Check sheet for the modelled part. Datum: model origin and axes. Units: mm. Face numbers are marked on the shaded views. A direction names the side the tool comes from. Round coordinates to 2 decimals unless told otherwise and drop trailing zeros. Loops run counter-clockwise (first coordinate to the right, second up) from the corner with the lowest first, then second, coordinate; pieces in that order, holes last. Notation, with made-up numbers: (40.25, 75) - (64.25, 75) arc R16 ccw to (64.25, 97) - close; hole circle Ø1 at (-16, 58). An arc over 180 degrees is marked (long way). Put each result on its own line as item: value.
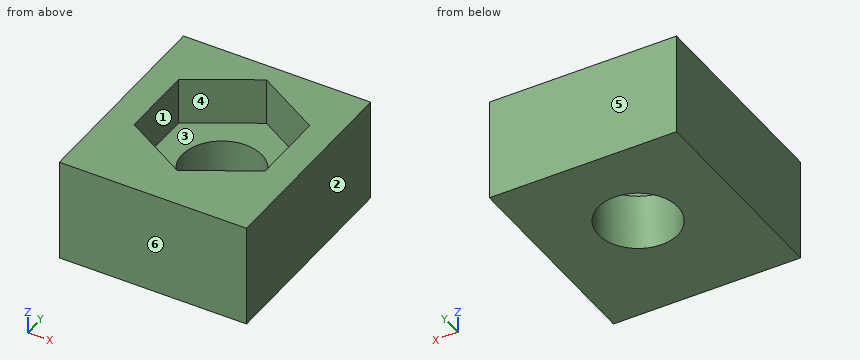
Autodesk Fusion 360 part; units mm, degrees
sketch "Sketch1" plane through (0, 0, 0) normal (0, 0, 1) x (1, 0, 0)
  line L0 (0, 0) -> (0, 8)
  line L1 (0, 0) -> (8, 0)
  line L2 (8, 0) -> (8, 8)
  line L3 (8, 8) -> (0, 8)
  dimension "d1" = 8
  dimension "d2" = 8
extrude "Extrude1" add sketch "Sketch1" along normal blind 2.4
sketch "Sketch2" plane through (0, 0, 2.4) normal (0, 0, 1) x (-1, 0, 0)
  line L0 (0, 0) -> (-8, 0)
  line L1 (-8, 0) -> (-8, -8)
  line L2 (-8, -8) -> (0, -8)
  line L3 (0, -8) -> (0, 0)
  line L4 (-8, -8) -> (0, 0)
  line L5 (-8, 0) -> (0, -8)
  line L6 (-6.8, -5.6166) -> (-4, -7.2332)
  line L7 (-4, -7.2332) -> (-1.2, -5.6166)
  line L8 (-1.2, -5.6166) -> (-1.2, -2.3834)
  line L9 (-1.2, -2.3834) -> (-4, -0.7668)
  line L10 (-4, -0.7668) -> (-6.8, -2.3834)
  line L11 (-6.8, -2.3834) -> (-6.8, -5.6166)
  point P0 (-4, -4)
  dimension "d5" = 2.8
extrude "Extrude2" add sketch "Sketch2" along normal blind 2 contours L0 L4 L5 L9 L10 | L3 L4 L5 L7 L8 L9 | L1 L4 L5 L6 L10 L11 | L2 L4 L5 L6 L7
sketch "Sketch3" plane through (0, 0, 2.4) normal (0, 0, 1) x (-1, 0, 0)
  line L0 (-6.8, -5.6166) -> (-4, -7.2332)
  line L1 (-4, -7.2332) -> (-1.2, -5.6166)
  line L2 (-1.2, -5.6166) -> (-1.2, -2.3834)
  line L3 (-1.2, -2.3834) -> (-4, -0.7668)
  line L4 (-4, -0.7668) -> (-6.8, -2.3834)
  line L5 (-6.8, -2.3834) -> (-6.8, -5.6166)
  circle A0 centre (-4, -4) radius 1.7
  dimension "d12" = 3.4
extrude "Extrude3" cut sketch "Sketch3" against normal blind 2.4 contours A0
sketch "Sketch4" plane through (0, 0, 0) normal (0, -1, 0) x (1, 0, 0)
  line L0 (0, 0) -> (8, 0)
  line L1 (8, 0) -> (8, 4.4)
  line L2 (8, 4.4) -> (0, 4.4)
  line L3 (0, 4.4) -> (0, 0)
  line L4 (8, 4.4) -> (0, 4.4)
  line L5 (0, 4.4) -> (0, 0)
  line L6 (0, 0) -> (8, 0)
  line L7 (8, 0) -> (8, 4.4)
extrude "Extrude4" add sketch "Sketch4" along normal blind 1
sketch "Sketch5" plane through (0, 0, 0) normal (-1, 0, 0) x (0, -1, 0)
  line L0 (-8, 0) -> (1, 0)
  line L1 (1, 0) -> (1, 4.4)
  line L2 (1, 4.4) -> (-8, 4.4)
  line L3 (-8, 4.4) -> (-8, 0)
Item 1: Tool access check on the marked faces 1 and 2. Record the directions out of +Z, -Z, +X, -X, +Y, -Y that give a thin tool (end or side, any length) a straight path to the whole face; none if there is none.
Filled sheet:
face 1: +Z
face 2: +Z, -Z, +X, +Y, -Y
Item 2: Section check D-D on z = 1.7. Enter the section's corners in (x, y), then the cut area to 3 significant figures.
Filled sheet:
outline: (0, -1) - (8, -1) - (8, 8) - (0, 8) - close; hole circle Ø3.4 at (4, 4)
area: 62.9 mm²
Item 3: Section check A-A on y = 4. Enter the section's corners in (x, z), then the cut area to 3 significant figures.
Filled sheet:
outline: (0, 0) - (2.3, 0) - (2.3, 2.4) - (1.2, 2.4) - (1.2, 4.4) - (0, 4.4) - close; (5.7, 0) - (8, 0) - (8, 4.4) - (6.8, 4.4) - (6.8, 2.4) - (5.7, 2.4) - close
area: 15.8 mm²
Item 4: Thickness scan on line 1 (X direction, y = 4, z = 0.75); line 2 (Y direction, x = 4, z = 0.9); line 3 (Z direction, x = 2.25, y = 3.5). Record the ranges inside material, lowest first. Write a range as from..to.
Filled sheet:
line 1: 0..2.3, 5.7..8
line 2: -1..2.3, 5.7..8
line 3: 0..2.4
Item 5: Release check for a two-part mould opening along Y. For the marked faces 3, 4, 5 and 6 record: +Y half, -Y half, draft (parallel to the pull), parting line (faces both ways), or undercut.
Filled sheet:
face 3: undercut
face 4: undercut
face 5: +Y half
face 6: -Y half
Item 6: Section check B-B on z = 4.15. Enter the section's corners in (x, y), then the cut area to 3 significant figures.
Filled sheet:
outline: (0, -1) - (8, -1) - (8, 8) - (0, 8) - close; hole (1.2, 2.38) - (4, 0.77) - (6.8, 2.38) - (6.8, 5.62) - (4, 7.23) - (1.2, 5.62) - close
area: 44.8 mm²
Item 7: Section check C-C on x = 3. Enter the section's corners in (y, z), then the cut area to 3 significant figures.
Filled sheet:
outline: (-1, 0) - (2.63, 0) - (2.63, 2.4) - (1.34, 2.4) - (1.34, 4.4) - (-1, 4.4) - close; (5.37, 0) - (8, 0) - (8, 4.4) - (6.66, 4.4) - (6.66, 2.4) - (5.37, 2.4) - close
area: 22.4 mm²
